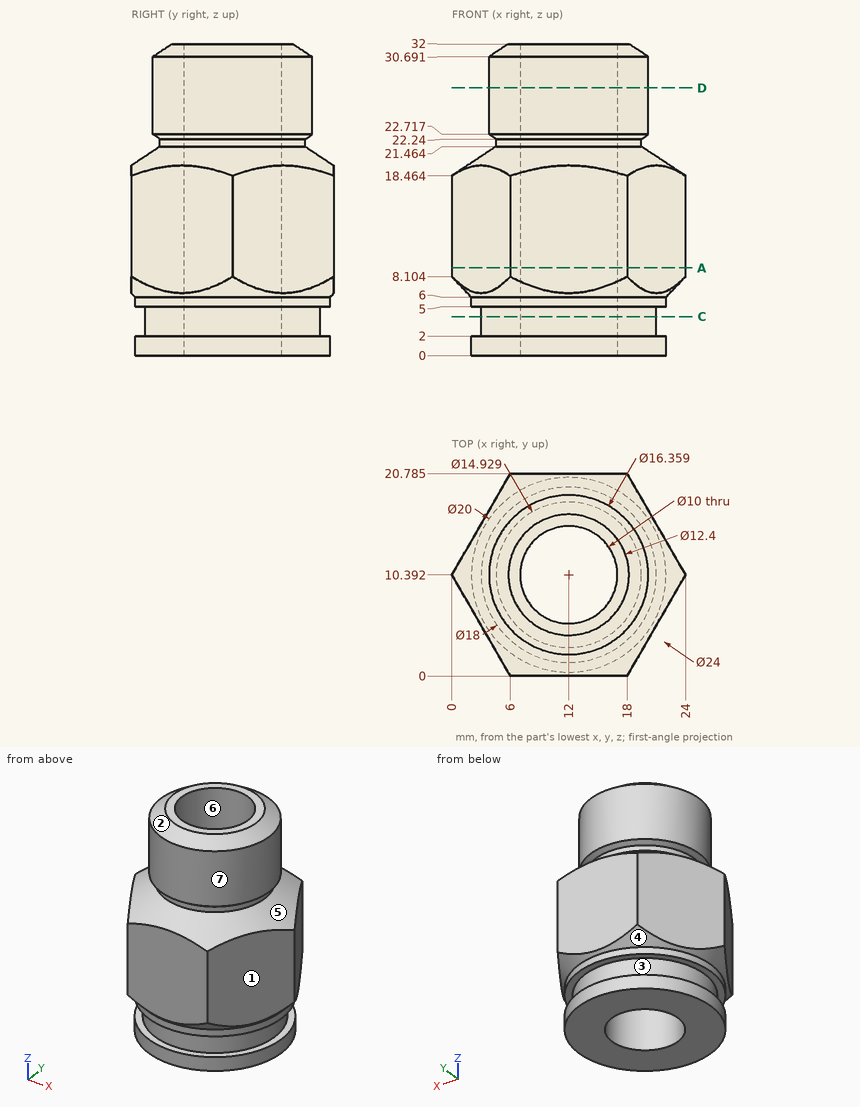
Here's the drawing with two shaded views (mm, measured from the low corner). I have some questions. A direction names the side the tool comes from. Coordinates: 2 decimals unless noted, no trailing zeros. Order: outer loops, then holes, each group sorted by start corner. A loop starts at its lowest first (then second) coordinate and runs counter-clockwise, first axis right, second up. Notation, with made-up numbers: M 42.25,10 L 67.25,10 A34 ccw 67.25,40 Z; hole C -9.5,89 d7. An arc over 180 degrees is marked long. Write item = value, one per line.
(1) Suppose I cut it at D-D on z = 27.5. Please give me the cut outline in (x, y).
Results are:
outline = C 12,10.39 d16.36; hole C 12,10.39 d10
(2) For pin 1 Ø5 at (x, y) = (17.5, 15.5) entering from -Z; pin 2 Ø5 at (x, z) = (14.5, 22) entering from -Y; pin 3 Ø1 at (y, z) = (12, 17) entering from +X; pin 4 Ø2 at (x, z) = (9.5, 22) entering from +Y, each with a flat end and sliding along its axis, tell me the tip position at first contact or that it passes through.
Results are:
pin_1 = 0
pin_2 = 0.22
pin_3 = 23.36
pin_4 = 18.37
(3) If we mould it in two halves opening along Z, with no side actions, what happens to the marked faces 1, 2, 3 and 4? For each: pulls with the +Z half, pulls with the -Z half, needs draft (parallel to the pull), parting line crosses it, or undercut.
Results are:
face_1 = needs draft
face_2 = pulls with the +Z half
face_3 = undercut
face_4 = pulls with the -Z half
(4) Suppose I cut it at C-C on z = 4. Please give me the cut outline in (x, y).
Results are:
outline = C 12,10.39 d18; hole C 12,10.39 d10
(5) For the marked faces 5, 6 and 7, which set-ups out of +Z, -Z, +X, -X, +Y, -Y let a thin tool reach every point of the face, with its end or its side?
Results are:
face_5 = none
face_6 = +Z, -Z
face_7 = +Z
(6) Suppose I cut it at A-A on z = 9. Please give me the cut outline in (x, y) (1 decimal).
Results are:
outline = M 0,10.4 L 6,0 L 18,0 L 24,10.4 L 18,20.8 L 6,20.8 Z; hole C 12,10.4 d10
(7) I need wall thicknesses on line 1 along Y through (x, z) = (12, 15) (1 decimal); line 2 along Y through (x, z) = (12, 24); line 3 along X through (y, z) = (10.25, 10). Which ranges of each line are inside material? Lowest first, please. Write a range as [from, to].
Results are:
line_1 = [0, 5.4], [15.4, 20.8]
line_2 = [2.21, 5.39], [15.39, 18.57]
line_3 = [0.08, 7], [17, 23.92]
